```python
from build123d import *

# Parameters (mm, degrees)
SKETCH001_W     = 139.6
SKETCH001_H     = 139.6
PAD_DEPTH       = 30
SKETCH002_W     = 130
SKETCH002_H     = 130
POCKET_DEPTH    = 25.2
SKETCH003_W     = 134.8
SKETCH003_H     = 134.8
POCKET001_DEPTH = 5
SKETCH004_R     = 5
SKETCH004_R_2   = 0.8255
PAD001_DEPTH    = 5
COPYSKETCH005_W = 70
COPYSKETCH005_H = 12.6
POCKET002_DEPTH = 5
SKETCH006_W     = 9
SKETCH006_H     = 5.5
POCKET003_DEPTH = 5
FILLET_R        = 2
FILLET001_R     = 2
FILLET002_R     = 2
FILLET003_R     = 2
FILLET004_R     = 1
FILLET005_R     = 1
FILLET006_R     = 1
FILLET007_R     = 3
FILLET008_R     = 3
FILLET009_R     = 3
FILLET010_R     = 3


with BuildPart() as part:
    # Sketch001 → Pad (new body)
    with BuildSketch(Plane.XY):
        Rectangle(SKETCH001_W, SKETCH001_H)
    extrude(amount=PAD_DEPTH)

    # Sketch002 (on Face6 of Pad) → Pocket (cut)
    with BuildSketch(Plane.XY.offset(30)):
        Rectangle(SKETCH002_W, SKETCH002_H)
    extrude(amount=-POCKET_DEPTH, mode=Mode.SUBTRACT)

    # Sketch003 (on Face5 of Pocket) → Pocket001 (cut)
    with BuildSketch(Plane.XY.offset(30)):
        Rectangle(SKETCH003_W, SKETCH003_H)
    extrude(amount=-POCKET001_DEPTH, mode=Mode.SUBTRACT)

    # Sketch004 (on Face16 of Pocket001) → Pad001 (join)
    with BuildSketch(Plane.XY.offset(4.8)):
        with Locations((-10, 36.18)):
            Circle(SKETCH004_R)
        with Locations((-10, 36.18)):
            Circle(SKETCH004_R_2, mode=Mode.SUBTRACT)
        with Locations((-10, -36.18)):
            Circle(SKETCH004_R)
        with Locations((-10, -36.18)):
            Circle(SKETCH004_R_2, mode=Mode.SUBTRACT)
    extrude(amount=PAD001_DEPTH)

    # CopySketch005 → Pocket002 (cut)
    with BuildSketch(Plane.YZ.offset(69.8)):
        with Locations((0, 23.7)):
            Rectangle(COPYSKETCH005_W, COPYSKETCH005_H)
    extrude(amount=-POCKET002_DEPTH, mode=Mode.SUBTRACT)

    # Sketch006 (on Face2 of Pocket002) → Pocket003 (cut)
    with BuildSketch(Plane(origin=(-69.8, 0, 0), x_dir=(0, -1, 0), z_dir=(-1, 0, 0))):
        with Locations((0, 27.25)):
            Rectangle(SKETCH006_W, SKETCH006_H)
    extrude(amount=-POCKET003_DEPTH, mode=Mode.SUBTRACT)

    # Fillet
    fillet_edges = [part.edges().sort_by_distance(p)[0] for p in [
        (65, -65, 14.9),
    ]]
    fillet(fillet_edges, radius=FILLET_R)

    # Fillet001
    fillet001_edges = [part.edges().sort_by_distance(p)[0] for p in [
        (65, 65, 14.9),
    ]]
    fillet(fillet001_edges, radius=FILLET001_R)

    # Fillet002
    fillet002_edges = [part.edges().sort_by_distance(p)[0] for p in [
        (-65, 65, 14.9),
    ]]
    fillet(fillet002_edges, radius=FILLET002_R)

    # Fillet003
    fillet003_edges = [part.edges().sort_by_distance(p)[0] for p in [
        (-65, -65, 14.9),
    ]]
    fillet(fillet003_edges, radius=FILLET003_R)

    # Fillet004
    fillet004_edges = [part.edges().sort_by_distance(p)[0] for p in [
        (-67.4, -67.4, 27.5),
    ]]
    fillet(fillet004_edges, radius=FILLET004_R)

    # Fillet005
    fillet005_edges = [part.edges().sort_by_distance(p)[0] for p in [
        (67.4, -67.4, 27.5),
    ]]
    fillet(fillet005_edges, radius=FILLET005_R)

    # Fillet006
    fillet006_edges = [part.edges().sort_by_distance(p)[0] for p in [
        (67.4, 67.4, 27.5),
    ]]
    fillet(fillet006_edges, radius=FILLET006_R)

    # Fillet007
    fillet007_edges = [part.edges().sort_by_distance(p)[0] for p in [
        (69.8, 69.8, 15),
    ]]
    fillet(fillet007_edges, radius=FILLET007_R)

    # Fillet008
    fillet008_edges = [part.edges().sort_by_distance(p)[0] for p in [
        (-69.8, 69.8, 15),
    ]]
    fillet(fillet008_edges, radius=FILLET008_R)

    # Fillet009
    fillet009_edges = [part.edges().sort_by_distance(p)[0] for p in [
        (-69.8, -69.8, 15),
    ]]
    fillet(fillet009_edges, radius=FILLET009_R)

    # Fillet010
    fillet010_edges = [part.edges().sort_by_distance(p)[0] for p in [
        (69.8, -69.8, 15),
    ]]
    fillet(fillet010_edges, radius=FILLET010_R)


solid = part.part
```
Model file for the job. Use its own axes, mm. A direction names the side the tool comes from. Coordinates: 2 decimals unless noted, no trailing zeros. Loops run counter-clockwise (first coordinate to the right, second up) from the corner with the lowest first, then second, coordinate; pieces in that order, holes last. Notation, with made-up numbers: M 31,4.5 L 62,4.5 A11 cw 62,17.5 Z; hole C 47,87 d11. An arc over 180 degrees is marked long. Use CSV: the item, a comma, the result in double quotes. Start each with the question number.
1. Probe probe 1 along Y at (x, z) = (-10, 8.5); probe 2 along X at (y, z) = (-62, 18). List the from-to ranges inside material, lowest first. Write a range as [from, to].
2. Tool access for faces 5 (the flat face through (67.4, -51, 28)), 6 (the flat face through (-69, -4.5, 27)), 7 (the flat face through (-1, -69.8, 15)): list every direction of +Z, -Z, +X, -X, +Y, -Y with a clear straight run to the whole face (end or side of a thin tool).
3. Band-saw the part on C-C, the plane y = 26. List the corners of the cut face in (x, z).
4. Band-saw the part on B-B, the plane z = 15.5. List the corners of the cut face in (x, y), then the cut area to 3 significant figures.
5. Flat gauge pins, fed straight in: pin 1 (5.5 mm diameter, centred on x = 67.5, y = 13, fed in from +Z); pin 2 (11 mm diameter, centred on x = -11, y = 35, fed in from +Z); pin 3 (1.3 mm diameter, centred on x = -10, y = 36.18, fed in from +Z). Where does each tip first touch, or does it go through?
6. Band-saw the part on A-A, the plane x = 28. List the corners of the cut face in (y, z).
7. Two-plate mould, pull along Y, no slides. Class faces 1 (the cylindrical face through (68.94, 68.9, 15.21)), 2 (the flat face through (-30, -66, 25)), 3 (the cylindrical face through (68.9, -68.94, 15.21)), 4 (the flat face through (-67.4, -36, 28)): pulls with the +Y half, pulls with the -Y half, needs draft (parallel to the pull), parting line crosses it, or undercut.
Entries:
1,probe 1,"y = [-69.8, -65], [-41.18, -37.01], [-35.35, -31.18], [31.18, 35.35], [37.01, 41.18], [65, 69.8]"
1,probe 2,"x = [-69.8, -65], [65, 69.8]"
2,face 5,"+Z"
2,face 6,"+Z, +X, -X"
2,face 7,"+Z, -Z, +X, -X, -Y"
3,outline,"M -69.8,0 L 69.8,0 L 69.8,17.4 L 65,17.4 L 65,4.8 L -65,4.8 L -65,25 L -67.4,25 L -67.4,30 L -69.8,30 Z"
4,outline,"M -69.8,-66.8 A3 ccw -66.8,-69.8 L 66.8,-69.8 A3 ccw 69.8,-66.8 L 69.8,66.8 A3 ccw 66.8,69.8 L -66.8,69.8 A3 ccw -69.8,66.8 Z; hole M -65,-63 A2 ccw -63,-65 L 63,-65 A2 ccw 65,-63 L 65,63 A2 ccw 63,65 L -63,65 A2 ccw -65,63 Z"
4,area,"2,580 mm2"
5,pin 1,"stops at z = 17.4"
5,pin 2,"stops at z = 9.8"
5,pin 3,"stops at z = 4.8"
6,outline,"M -69.8,0 L 69.8,0 L 69.8,30 L 67.4,30 L 67.4,25 L 65,25 L 65,4.8 L -65,4.8 L -65,25 L -67.4,25 L -67.4,30 L -69.8,30 Z"
7,face 1,"pulls with the +Y half"
7,face 2,"undercut"
7,face 3,"pulls with the -Y half"
7,face 4,"undercut"
